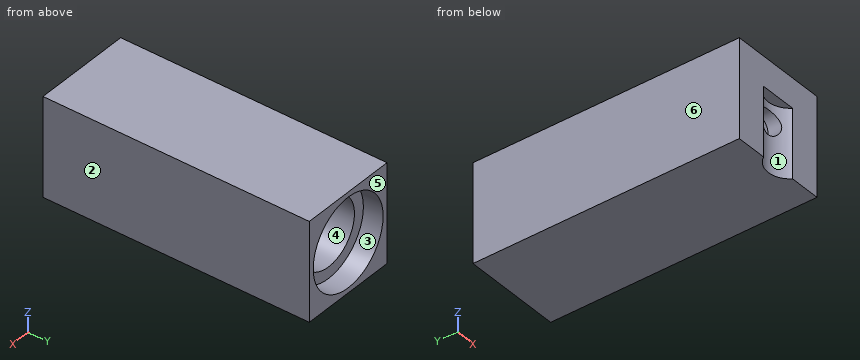
```python
from build123d import *

# Parameters (mm, degrees)
F0_W      = 10
F0_H      = 10
F1_DEPTH  = 27
F2_R      = 1.25
F3_DEPTH  = 25
F4_R      = 2.235
F5_DEPTH  = 25
F6_DEPTH  = 2
F7_R      = 3.35
F8_DEPTH  = 25
F9_R      = 4.5
F10_DEPTH = 2


with BuildPart() as f1:
    # F0 (on Front) → F1 (new body)
    with BuildSketch(Plane.XZ):
        Rectangle(F0_W, F0_H)
    extrude(amount=-F1_DEPTH)

    # F2 (on face) → F3 (cut)
    with BuildSketch(Plane.XZ):
        Circle(F2_R)
    extrude(amount=-F3_DEPTH, mode=Mode.SUBTRACT)

    # F4 (on Top) → F5 (cut)
    with BuildSketch(Plane.XY):
        with Locations((0, -1.235)):
            Circle(F4_R)
    extrude(amount=-F5_DEPTH, mode=Mode.SUBTRACT)

    # F4 (on Top) → F6 (cut)
    with BuildSketch(Plane.XY):
        with Locations((0, -1.235)):
            Circle(F4_R)
    extrude(amount=F6_DEPTH, mode=Mode.SUBTRACT)

    # F7 (on face) → F8 (cut)
    with BuildSketch(Plane(origin=(0, 27, 0), x_dir=(-1, 0, 0), z_dir=(0, 1, 0))):
        Circle(F7_R)
    extrude(amount=-F8_DEPTH, mode=Mode.SUBTRACT)

    # F9 (on face) → F10 (cut)
    with BuildSketch(Plane(origin=(0, 27, 0), x_dir=(-1, 0, 0), z_dir=(0, 1, 0))):
        Circle(F9_R)
    extrude(amount=-F10_DEPTH, mode=Mode.SUBTRACT)


solid = f1.part
```
CAD build for the part. Positions are in the model's coordinates, mm. Face numbers are marked on the shaded views. A direction names the side the tool comes from. Round coordinates to 2 decimals unless told otherwise and drop trailing zeros. Write each loop counter-clockwise with the first axis right and the second up, starting at its lowest first coordinate (ties: lowest second). Pieces come first, ordered by that corner, then holes. Notation, with made-up numbers: (89, 47.25) -> (129, 47.25) arc R12 ccw to (129, 68.25) -> close; hole circle Ø11 at (44, 85.5). An arc over 180 degrees is marked (long way). Answer in a Markdown table with one row per item. Add a question column.
Item 1: Saw through at A-A, the plane z = 0. Write the cut outline in (x, y) (3 decimals).
Item 2: Drill centre lines: line 1 (Z direction, x = 0, y = 26.3); line 2 (X direction, y = 1.7, z = 0); line 3 (Y direction, x = 2.75, z = 0.75). Where is each one in solid material? Low to high. Write a range as from..to.
Item 3: Mould opens along X. For the marked faces 3, 4, 5 and 6 say: pulls with the +X half, pulls with the -X half, needs draft (parallel to the pull), parting line crosses it, or undercut.
Item 4: Saw through at B-B, the plane x = 0. Write the cut outline in (y, z), then the cut area to 3 significant figures.
Item 5: Drop flat-ended pins along their axis: pin 1 Ø2 at (x, z) = (0, 0) entering from -Y; pin 2 Ø0.5 at (x, y) = (0, 0.5) entering from -Z; pin 3 Ø3.5 at (x, z) = (1, -1.5) entering from +Y; pin 4 Ø1 at (x, z) = (0.5, -3) entering from -Y. Give the stop position or say it passes through.
Item 6: Which spindle directions (+Z, -Z, +X, -X, +Y, -Y) get a long thin tool onto all of the face, cutting with end or side? Do the marked faces 1 and 2. Say none if no direction does.
Item 7: Saw through at D-D, the plane z = 2.25. Write the cut outline in (x, y).
Item 8: Saw through at C-C, the plane y = 5.5. Write the cut outline in (x, z).
Findings below:
| question | item | result |
|---|---|---|
| 1 | outline | (-5, 0) -> (-1.863, 0) arc R2.235 cw to (-1.25, 0.618) -> (-1.25, 2) -> (-3.35, 2) -> (-3.35, 25) -> (-4.5, 25) -> (-4.5, 27) -> (-5, 27) -> close; (1.25, 0.618) arc R2.235 cw to (1.863, 0) -> (5, 0) -> (5, 27) -> (4.5, 27) -> (4.5, 25) -> (3.35, 25) -> (3.35, 2) -> (1.25, 2) -> close |
| 2 | line 1 | z = -5..-4.5, 4.5..5 |
| 2 | line 2 | x = -5..-1.25, 1.25..5 |
| 2 | line 3 | y = 0..2 |
| 3 | face 3 | undercut |
| 3 | face 4 | undercut |
| 3 | face 5 | needs draft |
| 3 | face 6 | pulls with the -X half |
| 4 | outline | (0, 2) -> (1, 2) -> (1, 1.25) -> (2, 1.25) -> (2, 3.35) -> (25, 3.35) -> (25, 4.5) -> (27, 4.5) -> (27, 5) -> (0, 5) -> close; (1, -5) -> (27, -5) -> (27, -4.5) -> (25, -4.5) -> (25, -3.35) -> (2, -3.35) -> (2, -1.25) -> (1, -1.25) -> close |
| 4 | area | 88.4 mm^2 |
| 5 | pin 1 | passes through |
| 5 | pin 2 | stops at z = 2 |
| 5 | pin 3 | stops at y = 25 |
| 5 | pin 4 | stops at y = 0.76 |
| 6 | face 1 | -Z, -Y |
| 6 | face 2 | +Z, -Z, +X, +Y, -Y |
| 7 | outline | (-5, 0) -> (5, 0) -> (5, 27) -> (3.9, 27) -> (3.9, 25) -> (2.48, 25) -> (2.48, 2) -> (-2.48, 2) -> (-2.48, 25) -> (-3.9, 25) -> (-3.9, 27) -> (-5, 27) -> close |
| 8 | outline | (-5, -5) -> (5, -5) -> (5, 5) -> (-5, 5) -> close; hole circle Ø6.7 at (0, 0) |
